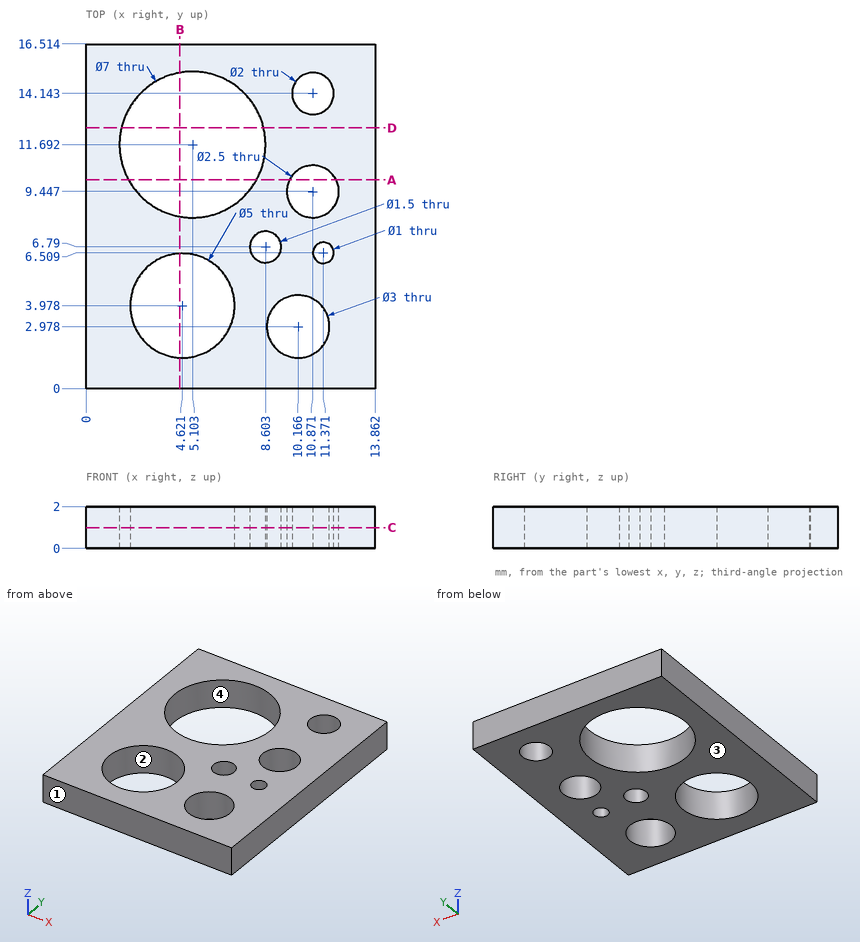
Could you check a few things on this drawing? It's one solid part, dimensions in mm from its lowest x, y, z. Coordinates: 2 decimals unless noted, no trailing zeros. Write each loop counter-clockwise with the first axis right and the second up, starting at its lowest first coordinate (ties: lowest second). Pieces come first, ordered by that corner, then holes.
1) If we section it at D-D (y = 12.5): List the corners of the cut face in (x, z) for me, plus the area to 3 significant figures.
Filled in:
outline: (0, 0) - (1.7, 0) - (1.7, 2) - (0, 2) - close; (8.51, 0) - (13.86, 0) - (13.86, 2) - (8.51, 2) - close
area: 14.1 mm2
2) I'm going to push flat-ended pins straight in: pin 1 (4.5 mm diameter, centred on x = 4.62, y = 3.98, fed in from -Z); pin 2 (5 mm diameter, centred on x = 10.17, y = 2.98, fed in from +Z). Where does each tip first touch, or does it pass through?
Filled in:
pin 1: passes through
pin 2: stops at z = 2
3) If we section it at C-C (z = 1): Count the separate pieces of the cut face and the enclosed holes in it, plus the area to 3 significant figures.
Filled in:
separate pieces: 1
enclosed holes: 7
area: 153 mm2
4) If I drill on line 1 (X direction, y = 14.75, z = 0.25) (1 decimal); line 2 (X direction, y = 2.5, z = 1.7) (1 decimal); line 3 (Y direction, x = 9, z = 1.1) (1 decimal), over which ranges is the centre line in solid material (lowest first)?
Filled in:
line 1: x = 0 to 3.4, 6.8 to 10.1, 11.7 to 13.9
line 2: x = 0 to 2.6, 6.6 to 8.7, 11.6 to 13.9
line 3: y = 0 to 2, 3.9 to 6.2, 7.4 to 16.5
5) If we section it at A-A (y = 10): List the corners of the cut face in (x, z) for me, plus the area to 3 significant figures.
Filled in:
outline: (0, 0) - (2.04, 0) - (2.04, 2) - (0, 2) - close; (8.17, 0) - (9.75, 0) - (9.75, 2) - (8.17, 2) - close; (11.99, 0) - (13.86, 0) - (13.86, 2) - (11.99, 2) - close
area: 11.0 mm2
6) If we section it at B-B (x = 4.5): List the corners of the cut face in (y, z) for me (1 decimal).
Filled in:
outline: (0, 0) - (1.5, 0) - (1.5, 2) - (0, 2) - close; (6.5, 0) - (8.2, 0) - (8.2, 2) - (6.5, 2) - close; (15.1, 0) - (16.5, 0) - (16.5, 2) - (15.1, 2) - close
7) Thinking about a two-plate mould opening in Y: for the marked faces 1, 2, 3 and 4, which applies, +Y half, -Y half, draft (parallel to the pull), parting line (faces both ways), or undercut?
Filled in:
face 1: -Y half
face 2: undercut
face 3: draft
face 4: undercut
